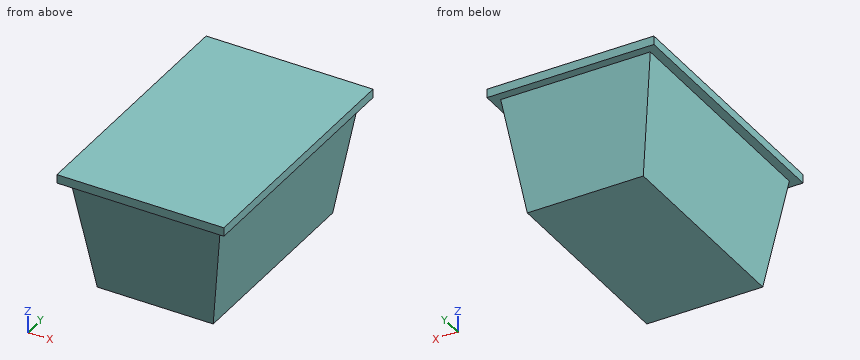
```python
from build123d import *

# Parameters (mm, degrees)
F1_DEPTH = 746.125
F3_DEPTH = 1270


with BuildPart() as f1:
    # F0 (on Front) → F1 (new body)
    with BuildSketch(Plane.XZ):
        Polygon((219.075, 76.2), (-219.075, 76.2), (-169.8625, -254), (169.8625, -254), align=None)
        Polygon((-244.475, 76.2), (-219.075, 76.2), (219.075, 76.2), (244.475, 76.2), (244.475, 101.6), (-244.475, 101.6), align=None)
    extrude(amount=F1_DEPTH)

    # F2 (on face) → F3 (cut)
    with BuildSketch(Plane.YZ.offset(244.475)):
        Polygon((-720.725, 76.2), (-746.125, 76.2), (-746.125, -258.798808), (-671.4998, -258.798808), align=None)
        Polygon((0, -255.167246), (0, 76.2), (-25.4, 76.2), (-74.6252, -255.167246), align=None)
    extrude(amount=-F3_DEPTH, mode=Mode.SUBTRACT)


solid = f1.part
```
For this review, take the finished solid that the model builds, in its own axes (mm). Coordinates: 2 decimals unless noted, no trailing zeros. Loops run counter-clockwise (first coordinate to the right, second up) from the corner with the lowest first, then second, coordinate; pieces in that order, holes last.
1. Add section A-A, the plane y = -203. Give the boundary of the cut face in (x, z) (1 decimal), then the cut area to 3 significant figures.
2. Add section D-D, the plane z = -202.5. Give the boundary of the cut face in (x, y).
3. Add section B-B, the plane x = -40.5. Give the boundary of the cut face in (y, z) (3 decimals), then the cut area to 3 significant figures.
4. Add section C-C, the plane z = -87.5. Give the boundary of the cut face in (x, y).
5. Insertion check: P1, Ø1, axis at y = -613, z = -155, coming from the -X side; P2, Ø10, axis at y = -160.5, z = -83.5, coming from the -X side; P3, Ø4, axis at y = -176, z = 3, coming from the -X side. Each pin has a flat end and moves straight along its axis. Give the tip position at first contact, or say it passes through.
6. For line 1 (Y direction, x = 52, z = 76); line 2 (Z direction, x = 225, y = -679); line 3 (Y direction, x = -5.5, z = 9), list the stretches that pass through material, from the lowest coordinate up.
Result:
1. outline: (-244.5, 76.2) - (-219.1, 76.2) - (-169.9, -254) - (169.9, -254) - (219.1, 76.2) - (244.5, 76.2) - (244.5, 101.6) - (-244.5, 101.6) - close
1. area: 141,000 mm2
2. outline: (-177.54, -679.77) - (177.54, -679.77) - (177.54, -66.8) - (-177.54, -66.8) - close
3. outline: (-746.125, 76.2) - (-720.725, 76.2) - (-672.205, -254) - (-74.452, -254) - (-25.4, 76.2) - (0, 76.2) - (0, 101.6) - (-746.125, 101.6) - close
3. area: 232,000 mm2
4. outline: (-194.68, -696.67) - (194.68, -696.67) - (194.68, -49.72) - (-194.68, -49.72) - close
5. P1: stops at x = -184.69
5. P2: stops at x = -196.02
5. P3: stops at x = -208.46
6. line 1: y = -720.7 to -25.43
6. line 2: z = 76.2 to 101.6
6. line 3: y = -710.85 to -35.38
